Design review of the part built by this model. Coordinates are the model's own, in mm. A direction names the side the tool comes from. Round coordinates to 2 decimals unless told otherwise and drop trailing zeros. Order: outer loops, then holes, each group sorted by start corner. A loop starts at its lowest first (then second) coordinate and runs counter-clockwise, first axis right, second up.
from build123d import *

# Parameters (mm, degrees)
SCHIZZO1_W                   = 700
SCHIZZO1_H                   = 470
ESTRUSIONE_ESTRUSIONE1_DEPTH = 15
SCHIZZO2_W                   = 40
SCHIZZO2_H                   = 470
ESTRUSIONE_ESTRUSIONE2_DEPTH = 40
RACCORDO1_R                  = 30
RACCORDO1_OF_SPECCHIA1_R     = 30


with BuildPart() as part:
    # Schizzo1 → Estrusione-Estrusione1 (new body)
    with BuildSketch(Plane.XY):
        Rectangle(SCHIZZO1_W, SCHIZZO1_H)
    extrude(amount=ESTRUSIONE_ESTRUSIONE1_DEPTH)

    # Schizzo2 → Estrusione-Estrusione2 (add)
    with BuildSketch(Plane.XY.offset(15)):
        with Locations((-315, 0)):
            Rectangle(SCHIZZO2_W, SCHIZZO2_H)
    estrusione_estrusione2 = extrude(amount=ESTRUSIONE_ESTRUSIONE2_DEPTH)

    # Raccordo1
    raccordo1_edges = [part.edges().sort_by_distance(p)[0] for p in [
        (-295, 0, 55),
    ]]
    fillet(raccordo1_edges, radius=RACCORDO1_R)

    # Specchia1: Estrusione-Estrusione2 across plane
    add(estrusione_estrusione2.mirror(Plane(origin=(0, 0, 0), x_dir=(0, 0, 1), z_dir=(1, 0, 0))))

    # Raccordo1 of Specchia1
    raccordo1_of_specchia1_edges = [part.edges().sort_by_distance(p)[0] for p in [
        (295, 0, 55),
    ]]
    fillet(raccordo1_of_specchia1_edges, radius=RACCORDO1_OF_SPECCHIA1_R)


solid = part.part
1) The part is to be moulded in two halves that separate along X. For faces 4 (the face through (-303.555, 3.29, 45.979)), 5 (the face through (350, -3, 7)), 6 (the face through (342, 3, 15)), 7 (the face through (-335, -3, 35)), say which applies: released by +X, released by -X, zero draft, split by the parting line, or undercut.
Results:
face 4: undercut
face 5: released by +X
face 6: zero draft
face 7: released by -X
2) Take a section at B-B on y = -43. Give the boundary of the cut face in (x, z), plus the area to 3 significant figures.
Results:
outline: (-350, 0) - (350, 0) - (350, 15) - (335, 15) - (335, 55) - (325, 55) arc R30 ccw to (295, 25) - (295, 15) - (-295, 15) - (-295, 25) arc R30 ccw to (-325, 55) - (-335, 55) - (-335, 15) - (-350, 15) - close
area: 13,300 mm2
3) For faces 1 (the face through (-343, 3, 15)), 2 (the face through (303.555, 3.29, 45.979)), 3 (the face through (335, -3, 35)), list the 3-axis set-ups (+Z, -Z, +X, -X, +Y, -Y) from which the entire face can be reached by the end or side of a thin tool; tool diameter is ignored.
Results:
face 1: +Z, -X, +Y, -Y
face 2: +Z, +Y, -Y
face 3: +Z, +X, +Y, -Y
4) Take a section at A-A on z = 38. Give the boundary of the cut face in (x, y), plus the area to 3 significant figures.
Results:
outline: (-335, -235) - (-297.96, -235) - (-297.96, 235) - (-335, 235) - close; (297.96, -235) - (335, -235) - (335, 235) - (297.96, 235) - close
area: 34,800 mm2
5) To check wall thickness, follow line 1 along X through (y, z) = (171, 22.5); line 2 along X through (y, z) = (76.5, 27.5); line 3 along Z through (x, y) = (246, 19.5). State the ranges of each line that lie inside material, in increasing order.
Results:
line 1: x = -335 to -295, 295 to 335
line 2: x = -335 to -295.1, 295.1 to 335
line 3: z = 0 to 15
6) Take a section at C-C on x = 69. Give the boundary of the cut face in (y, z), plus the area to 3 significant figures.
Results:
outline: (-235, 0) - (235, 0) - (235, 15) - (-235, 15) - close
area: 7,050 mm2
7) Clearance check with flat-ended pins moving along their axes: P1, Ø5, axis at x = 278, y = 90, coming from the +Z side; P2, Ø12, axis at y = 27, z = 44.5, coming from the -X side; P3, Ø2, axis at x = 180.5, y = 54, coming from the -Z side; P4, Ø5, axis at y = 56.5, z = 18.5, coming from the +X side. State where each tip first meets the part, or that it passes through.
Results:
P1: stops at z = 15
P2: stops at x = -335
P3: stops at z = 0
P4: stops at x = 335
